Read the model definition and answer for the solid it produces. Units are mm, in the model's axes. Face numbers are marked on the shaded views. Coordinates: 2 decimals unless noted, no trailing zeros. Loops run counter-clockwise (first coordinate to the right, second up) from the corner with the lowest first, then second, coordinate; pieces in that order, holes last. Notation, with made-up numbers: (28.5, -17) -> (40.5, -17) arc R22 ccw to (40.5, 21) -> close; hole circle Ø8 at (84, 39.5). An arc over 180 degrees is marked (long way). Answer as a JSON object with one key per item and string values. Group by question number.
Q1. Determine the mould class of the marked faces 1, 2 and 3 for opening direction X: released by +X, released by -X, zero draft, split by the parting line, or undercut.
Q2. The part is cut by section C-C on y = 0. Write down the section's boundary in (x, z).
Q3. Each of these flat-tipped pins is pushed along its axis until it touches: P1, Ø2.5, axis at y = 14, z = 2, coming from the +X side; P2, Ø0.9, axis at y = -13.5, z = 2, coming from the +X side; P3, Ø1.2, axis at y = -3.5, z = 7, coming from the -X side; P4, Ø2.5, axis at x = 0, y = 14, coming from the +Z side. Where does it stop, or does it pass through?
Q4. The part is cut by section B-B on y = 14. Write down the section's boundary in (x, z), and give its area (3 significant figures).
Q5. Straight lines are drawn through the part: line 1 along Z through (x, y) = (-3.5, -5.5); line 2 along X through (y, z) = (14, 3.6); line 3 along X through (y, z) = (-15.5, 1.25). For each, find the intervals that lie inside material, in ascending order. Write a range as [from, to].
Q6. The part is cut by section A-A on z = 5.5. Write down the section's boundary in (x, y), and give its area (3 significant figures).
Q7. The part is cut by section D-D on x = 29.5. Write down the section's boundary in (y, z).
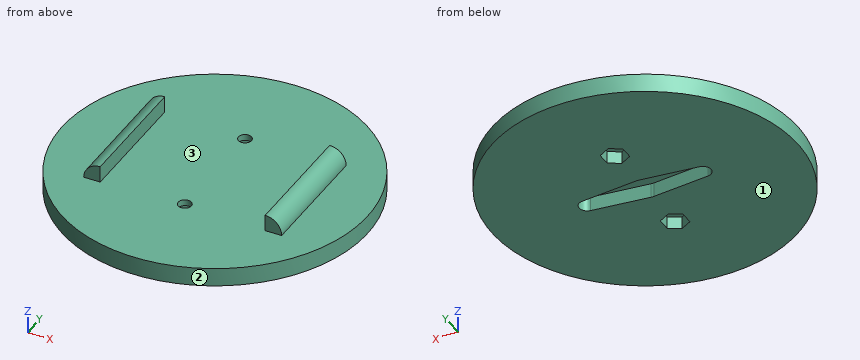
from build123d import *

# Parameters (mm, degrees)
F0_R      = 37
F1_DEPTH  = 4.5
F3_DEPTH  = 3.5
F5_DEPTH  = 15
F6_R      = 1.6
F7_DEPTH  = 4.501
F9_DEPTH  = 3
F11_ANGLE = 90


with BuildPart() as f1:
    # F0 (on Top) → F1 (new body)
    with BuildSketch(Plane.XY):
        Circle(F0_R)
    extrude(amount=F1_DEPTH)

    # F2 (on face) → F3 (cut)
    with BuildSketch(Plane(origin=(0, 0, 0), x_dir=(1, 0, 0), z_dir=(0, 0, -1))):
        with BuildLine():
            ThreePointArc((3.4798527268, -0.375), (3.4949595522, -0.1877704134), (3.5, 0))
            ThreePointArc((3.5, 0), (3.4949595522, 0.1877704134), (3.4798527268, 0.375))
            ThreePointArc((3.4798527268, 0.375), (2.3385358667, 2.604083332), (0, 3.5))
            ThreePointArc((0, 3.5), (-2.3385358667, 2.604083332), (-3.4798527268, 0.375))
            ThreePointArc((-3.4798527268, 0.375), (-3.5, 0), (-3.4798527268, -0.375))
            ThreePointArc((-3.4798527268, -0.375), (0, -3.5), (3.4798527268, -0.375))
        make_face()
        with BuildLine():
            ThreePointArc((0, 3.5), (2.3385358667, 2.604083332), (3.4798527268, 0.375))
            Line((3.4798527268, 0.375), (1.9884872724, 14.2142857143))
            ThreePointArc((1.9884872724, 14.2142857143), (1.9971197441, 14.1072973791), (2, 14))
            ThreePointArc((2, 14), (1.4142135624, 12.5857864376), (0, 12))
            Line((0, 12), (0, 3.5))
        make_face()
        with BuildLine():
            Line((1.9884872724, -14.2142857143), (3.4798527268, -0.375))
            ThreePointArc((3.4798527268, -0.375), (0, -3.5), (-3.4798527268, -0.375))
            Line((-3.4798527268, -0.375), (-1.9884872724, -14.2142857143))
            ThreePointArc((-1.9884872724, -14.2142857143), (-0.1072973791, -12.0028802559), (2, -14))
            ThreePointArc((2, -14), (1.9971197441, -14.1072973791), (1.9884872724, -14.2142857143))
        make_face()
        with BuildLine():
            ThreePointArc((-3.4798527268, 0.375), (-2.3385358667, 2.604083332), (0, 3.5))
            Line((0, 3.5), (0, 12))
            ThreePointArc((0, 12), (-1.4880476183, 12.6636937904), (-1.9884872724, 14.2142857143))
            Line((-1.9884872724, 14.2142857143), (-3.4798527268, 0.375))
        make_face()
        with BuildLine():
            ThreePointArc((2, 14), (1.9971197441, 14.1072973791), (1.9884872724, 14.2142857143))
            ThreePointArc((1.9884872724, 14.2142857143), (0, 16), (-1.9884872724, 14.2142857143))
            ThreePointArc((-1.9884872724, 14.2142857143), (-1.4880476183, 12.6636937904), (0, 12))
            ThreePointArc((0, 12), (1.4142135624, 12.5857864376), (2, 14))
        make_face()
        with BuildLine():
            ThreePointArc((-1.9884872724, -14.2142857143), (0, -16), (1.9884872724, -14.2142857143))
            ThreePointArc((1.9884872724, -14.2142857143), (1.9971197441, -14.1072973791), (2, -14))
            ThreePointArc((2, -14), (-0.1072973791, -12.0028802559), (-1.9884872724, -14.2142857143))
        make_face()
    extrude(amount=-F3_DEPTH, mode=Mode.SUBTRACT)

    # F4 (on Right) → F5 (join, symmetric)
    with BuildSketch(Plane.YZ):
        with BuildLine():
            ThreePointArc((-20, 8.5), (-22.8284271247, 7.3284271247), (-24, 4.5))
            Line((-24, 4.5), (-20, 4.5))
            Line((-20, 4.5), (-20, 8.5))
        make_face()
        with BuildLine():
            Line((20, 8.5), (20, 4.5))
            Line((20, 4.5), (24, 4.5))
            ThreePointArc((24, 4.5), (22.8284271247, 7.3284271247), (20, 8.5))
        make_face()
    extrude(amount=F5_DEPTH, both=True)

    # F6 (on face) → F7 (cut, through all)
    with BuildSketch(Plane.XY.offset(4.5)):
        with Locations((-14, 0)):
            Circle(F6_R)
        with Locations((14, 0)):
            Circle(F6_R)
    extrude(amount=-F7_DEPTH, mode=Mode.SUBTRACT)

    # F8 (on face) → F9 (cut)
    with BuildSketch(Plane(origin=(0, 0, 0), x_dir=(1, 0, 0), z_dir=(0, 0, -1))):
        Polygon((12.4122867597, 2.75), (10.8245735195, 0), (12.4122867597, -2.75), (15.5877132403, -2.75), (17.1754264805, 0), (15.5877132403, 2.75), align=None)
        Polygon((-12.4122867597, -2.75), (-10.8245735195, 0), (-12.4122867597, 2.75), (-15.5877132403, 2.75), (-17.1754264805, 0), (-15.5877132403, -2.75), align=None)
    extrude(amount=-F9_DEPTH, mode=Mode.SUBTRACT)


with BuildPart() as f1_1:
    # F11: moved
    add(f1.part.rotate(Axis((0, 0, 35.3244128637), (0, 0, 1)), F11_ANGLE))


solid = f1_1.part
Final values:
{
 "1": {"face 1": "zero draft", "face 2": "split by the parting line", "face 3": "undercut"},
 "2": {"outline": "(-37, 0) -> (-16, 0) -> (-16, 3.5) -> (16, 3.5) -> (16, 0) -> (37, 0) -> (37, 4.5) -> (24, 4.5) arc R4 ccw to (20, 8.5) -> (20, 4.5) -> (-20, 4.5) -> (-20, 8.5) arc R4 ccw to (-24, 4.5) -> (-37, 4.5) -> close"},
 "3": {"P1": "stops at x = 34.73", "P2": "stops at x = 34.62", "P3": "stops at x = -23.52", "P4": "passes through"},
 "4": {"outline": "(-34.25, 0) -> (-2.75, 0) -> (-2.75, 3) -> (-1.6, 3) -> (-1.6, 4.5) -> (-20, 4.5) -> (-20, 8.5) arc R4 ccw to (-24, 4.5) -> (-34.25, 4.5) -> close; (1.6, 3) -> (2.75, 3) -> (2.75, 0) -> (34.25, 0) -> (34.25, 4.5) -> (24, 4.5) arc R4 ccw to (20, 8.5) -> (20, 4.5) -> (1.6, 4.5) -> close", "area": "312 mm2"},
 "5": {"line 1": "z = [0, 4.5]", "line 2": "x = [-34.25, -1.6], [1.6, 34.25]", "line 3": "x = [-33.6, -2.75], [2.75, 33.6]"},
 "6": {"outline": "(-23.87, -15) -> (-20, -15) -> (-20, 15) -> (-23.87, 15) -> close; (20, -15) -> (23.87, -15) -> (23.87, 15) -> (20, 15) -> close", "area": "232 mm2"},
 "7": {"outline": "(-22.33, 0) -> (22.33, 0) -> (22.33, 4.5) -> (-22.33, 4.5) -> close"}
}
